```python
from build123d import *

# Parameters (mm, degrees)
SKETCH1_W               = 124.46
SKETCH1_H               = 57.404
BOSS_EXTRUDE1_DEPTH     = 2.54
CUT_EXTRUDE1_START      = -57.404
CUT_EXTRUDE1_DEPTH      = 57.404
CUT_EXTRUDE2_DEPTH      = 138.083778822
CUT_EXTRUDE2_DEPTH_BACK = 138.083778822
SKETCH5_W               = 2.54
SKETCH5_H               = 57.404
BOSS_EXTRUDE2_DEPTH     = 6.35
SKETCH7_W               = 2.54
SKETCH7_H               = 57.404
BOSS_EXTRUDE3_DEPTH     = 6.35


# Read off the part's stored shape, not the designer's step: Cut-Extrude1
with BuildPart() as part:
    # Sketch1 → Boss-Extrude1 (new body)
    with BuildSketch(Plane(origin=(0, 0, 0), x_dir=(1, 0, 0), z_dir=(0, 1, 0))):
        with Locations((62.23, 28.702)):
            Rectangle(SKETCH1_W, SKETCH1_H)
    extrude(amount=BOSS_EXTRUDE1_DEPTH)

    # Cut-Extrude1 outline → Cut-Extrude1 (cut)
    with BuildSketch(Plane.XY.offset(CUT_EXTRUDE1_START)):
        with BuildLine():
            Line((0, 2.54), (0, 0.035695157))
            ThreePointArc((0, 0.035695157), (0.738676689, 1.801323311), (2.504304843, 2.54))
            Line((2.504304843, 2.54), (0, 2.54))
        make_face()
    extrude(amount=CUT_EXTRUDE1_DEPTH, mode=Mode.SUBTRACT)

    # Sketch4 → Cut-Extrude2 (cut, two sides: drawn at the far end of the back side and taken through both)
    with BuildSketch(Plane.XY.offset(-CUT_EXTRUDE2_DEPTH_BACK)):
        with BuildLine():
            Line((-137.051831338, 2.54), (121.92, 2.54))
            ThreePointArc((121.92, 2.54), (123.716051224, 1.796051224), (124.46, 0))
            Line((124.46, 0), (124.46, -258.971831338))
            Line((124.46, -258.971831338), (490.701476151, 107.269644813))
            Line((490.701476151, 107.269644813), (229.189644813, 368.781476151))
            Line((229.189644813, 368.781476151), (-137.051831338, 2.54))
        make_face()
    extrude(amount=CUT_EXTRUDE2_DEPTH + CUT_EXTRUDE2_DEPTH_BACK, mode=Mode.SUBTRACT)

    # Sketch5 → Boss-Extrude2 (add)
    with BuildSketch(Plane.XZ):
        with Locations((1.27, -28.702)):
            Rectangle(SKETCH5_W, SKETCH5_H)
    extrude(amount=BOSS_EXTRUDE2_DEPTH)

    # Sketch7 → Boss-Extrude3 (add)
    with BuildSketch(Plane.XZ):
        with Locations((123.19, -28.702)):
            Rectangle(SKETCH7_W, SKETCH7_H)
    extrude(amount=BOSS_EXTRUDE3_DEPTH)


solid = part.part
```
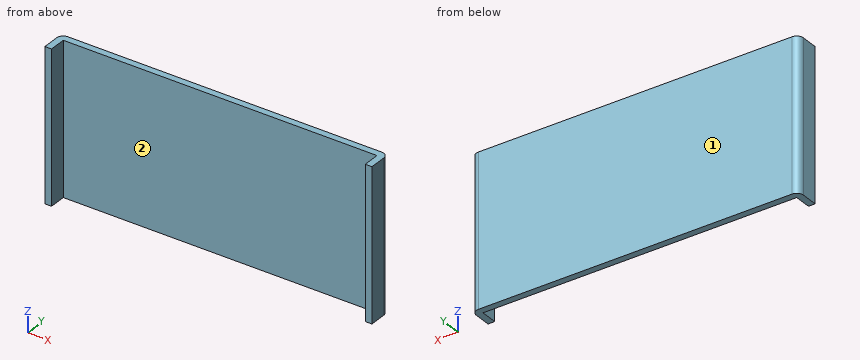
The model under review builds one solid part; all positions refer to its coordinate system, in mm. Face numbers are marked on the shaded views. Round coordinates to 2 decimals unless told otherwise and drop trailing zeros. Order: outer loops, then holes, each group sorted by start corner. A loop starts at its lowest first (then second) coordinate and runs counter-clockwise, first axis right, second up. Notation, with made-up numbers: (52, 61.25) - (71, 61.25) arc R15 cw to (71, 73.25) - close; hole circle Ø10 at (87.5, 36). An arc over 180 degrees is marked (long way). Answer in a Markdown table with one row per item.
(1) Take a section at B-B on z = -4.5. Write out the cut boundary in (x, y).
Result set:
| item | result |
|---|---|
| outline | (0, -6.35) - (2.54, -6.35) - (2.54, 0) - (121.92, 0) - (121.92, -6.35) - (124.46, -6.35) - (124.46, 0) arc R2.54 ccw to (121.92, 2.54) - (2.5, 2.54) arc R2.52 ccw to (0, 0.04) - close |
(2) Take a section at A-A on y = -3. Write out the cut boundary in (x, z), plus the area to 3 significant figures.
Result set:
| item | result |
|---|---|
| outline | (0, -57.4) - (2.54, -57.4) - (2.54, 0) - (0, 0) - close; (121.92, -57.4) - (124.46, -57.4) - (124.46, 0) - (121.92, 0) - close |
| area | 292 mm2 |
(3) Clearance check with flat-ended pins moving along their axes: P1, Ø5, axis at x = 36, z = -15.5, coming from the -Y side; P2, Ø5, axis at x = 31, y = -3.5, coming from the +Z side. State where each tip first meets the part, or that it passes through.
Result set:
| item | result |
|---|---|
| P1 | stops at y = 0 |
| P2 | passes through |
(4) Take a section at C-C on x = 53. Write out the cut boundary in (y, z), plus the area to 3 significant figures.
Result set:
| item | result |
|---|---|
| outline | (0, -57.4) - (2.54, -57.4) - (2.54, 0) - (0, 0) - close |
| area | 146 mm2 |
(5) For line 1 (X direction, y = -1.25, z = -23); line 2 (Y direction, x = 91.5, z = -46); line 3 (X direction, y = 0.25, z = -3), list the stretches that pass through material, from the lowest coordinate up. Write a range as from..to.
Result set:
| item | result |
|---|---|
| line 1 | x = 0..2.54, 121.92..124.46 |
| line 2 | y = 0..2.54 |
| line 3 | x = 0.01..124.45 |
(6) Mouldability with a two-part tool opening along X and no side actions: class the marked faces 1 and 2 as released by +X, released by -X, zero draft, split by the parting line, or undercut.
Result set:
| item | result |
|---|---|
| face 1 | zero draft |
| face 2 | undercut |
